from build123d import *

# Parameters (mm, degrees)
SKETCH1_W           = 9
SKETCH1_H           = 25.4
BOSS_EXTRUDE1_DEPTH = 12
SKETCH2_W           = 5
SKETCH2_H           = 3
CUT_EXTRUDE1_DEPTH  = 30.498474537
SKETCH4_W           = 5.5
SKETCH4_H           = 8
CUT_EXTRUDE2_DEPTH  = 22
SKETCH7_W           = 5.5
SKETCH7_H           = 8
SKETCH7_R           = 2.235
BOSS_EXTRUDE3_DEPTH = 7.8
SKETCH8_R           = 2.235
BOSS_EXTRUDE4_DEPTH = 3.4162


with BuildPart() as part:
    # Sketch1 → Boss-Extrude1 (new body)
    with BuildSketch(Plane(origin=(0, 0, 0), x_dir=(1, 0, 0), z_dir=(0, 1, 0))):
        with Locations((-4.5, 12.7)):
            Rectangle(SKETCH1_W, SKETCH1_H)
    extrude(amount=BOSS_EXTRUDE1_DEPTH)

    # Sketch2 → Cut-Extrude1 (cut, through all)
    with BuildSketch(Plane(origin=(0, 12, 0), x_dir=(1, 0, 0), z_dir=(0, 1, 0))):
        with Locations((-4.5, 12.7)):
            Rectangle(SKETCH2_W, SKETCH2_H)
    extrude(amount=-CUT_EXTRUDE1_DEPTH, mode=Mode.SUBTRACT)

    # Sketch4 → Cut-Extrude2 (cut)
    with BuildSketch(Plane(origin=(0, 0, -25.4), x_dir=(-1, 0, 0), z_dir=(0, 0, -1))):
        with Locations((4.5, 6)):
            Rectangle(SKETCH4_W, SKETCH4_H)
    extrude(amount=-CUT_EXTRUDE2_DEPTH, mode=Mode.SUBTRACT)

    # Sketch7 → Boss-Extrude3 (add)
    with BuildSketch(Plane(origin=(0, 0, -3.4), x_dir=(-1, 0, 0), z_dir=(0, 0, -1))):
        with Locations((4.5, 6)):
            Rectangle(SKETCH7_W, SKETCH7_H)
        with Locations(Location((4.5, 6, 0), (0, 0, 180))):
            Circle(SKETCH7_R, mode=Mode.SUBTRACT)
    extrude(amount=BOSS_EXTRUDE3_DEPTH)

    # Sketch8 → Boss-Extrude4 (add)
    with BuildSketch(Plane(origin=(0, 0, -3.4), x_dir=(-1, 0, 0), z_dir=(0, 0, -1))):
        with Locations(Location((4.5, 6, 0), (0, 0, 180))):
            Circle(SKETCH8_R)
    extrude(amount=BOSS_EXTRUDE4_DEPTH)


solid = part.part
Design review of the part built by this model. Coordinates are the model's own, in mm. A direction names the side the tool comes from. Give positions to 0.01 mm unless a question says otherwise; leave off trailing zeros. Order: outer loops, then holes, each group sorted by start corner. A loop starts at its lowest first (then second) coordinate and runs counter-clockwise, first axis right, second up. Notation, with made-up numbers: (-23, 41) - (6, 41) arc R18 ccw to (6, 58) - close; hole circle Ø2 at (57.25, -38.75). An arc over 180 degrees is marked (long way). Write item = value, one per line. Start each with the question number.
Q1. Tool access review of faces 5 (the face through (-5, 0, -10)), 6 (the face through (-7, 1, -13)), 7 (the face through (-7.25, 6, -18)): name each direction out of +Z, -Z, +X, -X, +Y, -Y from which nothing blocks a thin tool from reaching the whole face with its end or side.
Q2. We need section D-D on y = 9.75. State the section outline as (x, z) points.
Q3. To check wall thickness, follow L1, parallel to X at y = 6.75, z = -19.75; L2, parallel to X at y = 6, z = -7.9 (3 decimals); L3, parallel to Y at x = -4.5, z = -9.3 (3 decimals). State the ranges of each line that lie inside material, in increasing order. Write a range as from..to.
Q4. We need section B-B on z = -22. State the section outline as (x, y) points.
Q5. Clearance check with flat-ended pins moving along their axes: pin 1 Ø5 at (x, z) = (-5.5, -11) entering from -Y; pin 2 Ø1.6 at (x, y) = (-4.5, 4) entering from -Z; pin 3 Ø2.5 at (x, y) = (-4.5, 6) entering from -Z. State where each tip first meets the part, or that it passes through.
Q6. Mouldability with a two-part tool opening along Z and no side actions: class faces 1 (the face through (-5, 1, -14.2)), 2 (the face through (-9, 6, -13)), 3 (the face through (-5, 6, 0)), 4 (the face through (-1.56, 5.92, -25.4)) as released by +Z, released by -Z, zero draft, split by the parting line, or undercut.
Q7. We need section A-A on x = -4.5. State the section outline as (y, z) points (3 decimals).
Q8. We need section C-C on y = 1.75. State the section outline as (x, z) points.
Working result:
q1.face_5 = +Z, -Z, +X, -X, -Y
q1.face_6 = +Y, -Y
q1.face_7 = -Z
q2.outline = (-9, -25.4) - (-7.25, -25.4) - (-7.25, -11.2) - (-1.75, -11.2) - (-1.75, -25.4) - (0, -25.4) - (0, 0) - (-9, 0) - close
q3.L1 = -9..-7.25, -1.75..0
q3.L2 = -9..-6.735, -2.265..0
q3.L3 = 0..3.765, 8.235..12
q4.outline = (-9, 0) - (0, 0) - (0, 12) - (-9, 12) - close; hole (-7.25, 2) - (-1.75, 2) - (-1.75, 10) - (-7.25, 10) - close
q5.pin_1 = 0
q5.pin_2 = -11.2
q5.pin_3 = -6.82
q6.face_1 = undercut
q6.face_2 = zero draft
q6.face_3 = released by +Z
q6.face_4 = released by -Z
q7.outline = (0, -25.4) - (2, -25.4) - (2, -14.2) - (0, -14.2) - close; (0, -11.2) - (3.765, -11.2) - (3.765, -6.816) - (8.235, -6.816) - (8.235, -11.2) - (12, -11.2) - (12, 0) - (0, 0) - close; (10, -25.4) - (12, -25.4) - (12, -14.2) - (10, -14.2) - close
q8.outline = (-9, -25.4) - (0, -25.4) - (0, 0) - (-9, 0) - close; hole (-7, -14.2) - (-2, -14.2) - (-2, -11.2) - (-7, -11.2) - close
